Design review of the part shown in the three views and the two pictorial views. Dimensions are in mm from the part's minimum x, y and z. Round coordinates to 2 decimals unless told otherwise and drop trailing zeros. Loops run counter-clockwise (first coordinate to the right, second up) from the corner with the lowest first, then second, coordinate; pieces in that order, holes last. Notation, with made-up numbers: M -30.5,-12.75 L 14.5,-12.75 A14 cw 14.5,10.25 Z; hole C -9.75,-21 d11. An arc over 180 degrees is marked long. One line per question, with ' | ' between items.
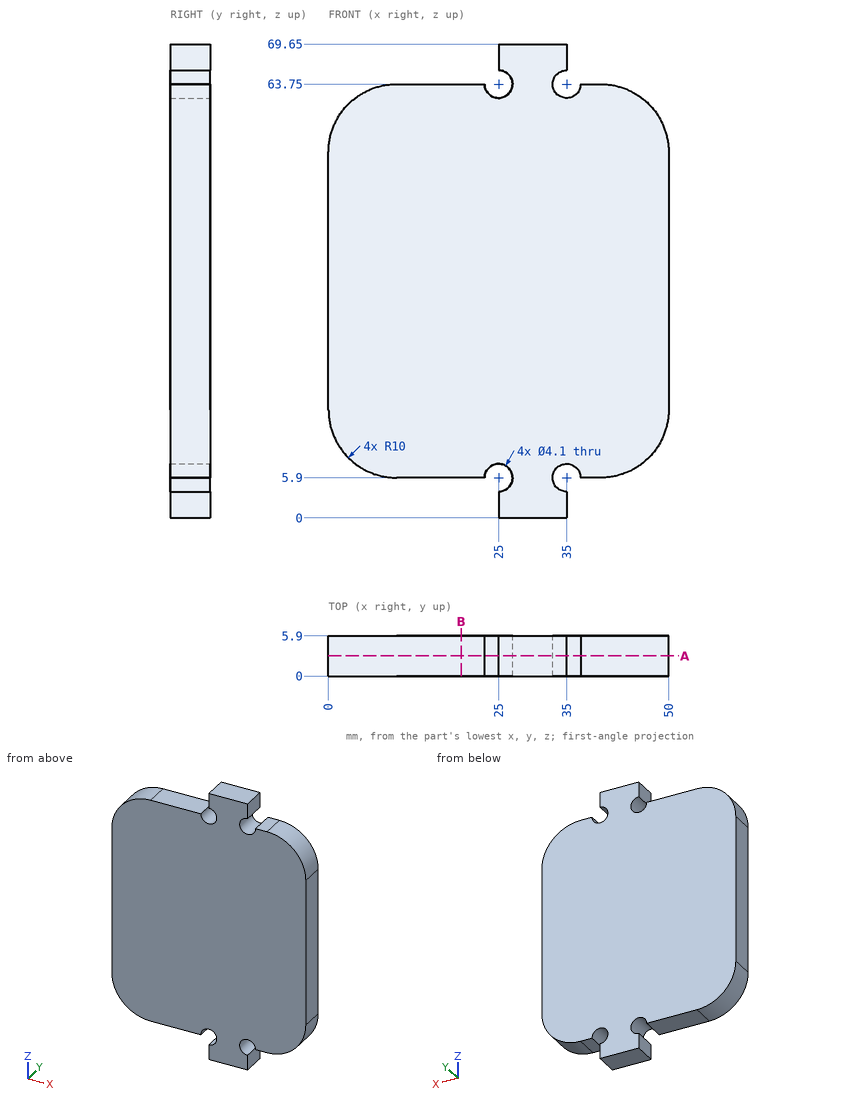
1) Insertion check: P1, Ø3, axis at x = 38, y = 2, coming from the +Z side; P2, Ø3.5, axis at x = 25, z = 5.9, coming from the -Y side; P3, Ø1.9, axis at y = 4, z = 2.5, coming from the -X side; P4, Ø1.2, axis at y = 2, z = 2, coming from the +X side. Each pin has a flat end and moves straight along its axis. Give the tip position at first contact, or say it passes through.
Output values:
P1: stops at z = 63.75 | P2: passes through | P3: stops at x = 25 | P4: stops at x = 35
2) Add section A-A on y = 2.95. State the section outline as (x, z) points.
Output values:
outline: M 0,15.9 A10 ccw 10,5.9 L 22.95,5.9 A2.05 cw long 25,3.85 L 25,0 L 35,0 L 35,3.85 A2.05 cw long 37.05,5.9 L 40,5.9 A10 ccw 50,15.9 L 50,53.75 A10 ccw 40,63.75 L 37.05,63.75 A2.05 cw long 35,65.8 L 35,69.65 L 25,69.65 L 25,65.8 A2.05 cw long 22.95,63.75 L 10,63.75 A10 ccw 0,53.75 Z
3) Add section B-B on x = 19.5. State the section outline as (y, z) points.
Output values:
outline: M 0,5.9 L 5.9,5.9 L 5.9,63.75 L 0,63.75 Z
4) For line 1 (X direction, y = 3, z = 62.5); line 2 (Z direction, x = 19.5, y = 3.45), list the stretches that pass through material, from the lowest coordinate up.
Output values:
line 1: x = 5.16 to 23.38, 26.62 to 33.38, 36.62 to 44.84 | line 2: z = 5.9 to 63.75
